```python
from build123d import *

# Parameters (mm, degrees)
SKETCH_1_R          = 12.2
EXTRUDE_1_DEPTH     = 30.8
SKETCH_3_R          = 3.15
EXTRUDE_2_DEPTH     = 2.1
FILLET_1_R          = 0.5
SKETCH_4_R          = 3.225
EXTRUDE_3_DEPTH     = 1.7
SKETCH_6_R          = 1
EXTRUDE_4_DEPTH     = 10
SKETCH_7_R          = 1.1
CUT_EXTRUDE_2_DEPTH = 3


with BuildPart() as part:
    # 草图1 → 凸台-拉伸1 (new body)
    with BuildSketch(Plane(origin=(0, 0, 0), x_dir=(0, 0, -1), z_dir=(1, 0, 0))):
        with Locations(Location((0, 0, 0), (0, 0, 180))):
            Circle(SKETCH_1_R)
    extrude(amount=EXTRUDE_1_DEPTH)

    # 草图3 → 凸台-拉伸2 (add)
    with BuildSketch(Plane(origin=(30.8, 0, 0), x_dir=(0, 0, -1), z_dir=(1, 0, 0))):
        Circle(SKETCH_3_R)
    extrude(amount=EXTRUDE_2_DEPTH)

    # 圆角1
    fillet_1_edges = [part.edges().sort_by_distance(p)[0] for p in [
        (32.9, 0, 3.15),
    ]]
    fillet(fillet_1_edges, radius=FILLET_1_R)

    # 草图4 → 凸台-拉伸3 (add)
    with BuildSketch(Plane.ZY):
        Circle(SKETCH_4_R)
    extrude(amount=EXTRUDE_3_DEPTH)

    # 草图6 → 凸台-拉伸4 (add)
    with BuildSketch(Plane.ZY):
        Circle(SKETCH_6_R)
    extrude(amount=EXTRUDE_4_DEPTH)

    # 草图7 → 切除-拉伸2 (cut)
    with BuildSketch(Plane.ZY):
        with Locations((8.5, 0)):
            Circle(SKETCH_7_R)
        with Locations((-8.5, 0)):
            Circle(SKETCH_7_R)
    extrude(amount=-CUT_EXTRUDE_2_DEPTH, mode=Mode.SUBTRACT)


solid = part.part
```
Geometry check sheet. Reference: the model listing, model coordinates, mm. A direction names the side the tool comes from. Give positions to 0.01 mm unless a question says otherwise; leave off trailing zeros. Order: outer loops, then holes, each group sorted by start corner. A loop starts at its lowest first (then second) coordinate and runs counter-clockwise, first axis right, second up.
1. Release check for a two-part mould opening along Y. For faces 4 (the face through (3, 0, -9)), 5 (the face through (-0.84, -3.15, -0.7)), 6 (the face through (-10, 0, 0)) record: pulls with the +Y half, pulls with the -Y half, needs draft (parallel to the pull), parting line crosses it, or undercut.
2. Section check C-C, the plane x = 2. Enter the section's corners in (y, z), and give its area (3 significant figures).
3. Access from +Z, -Z, +X, -X, +Y, -Y to the whole of each face (thin tool, end or side, straight path). Record for faces 1 (the face through (1.479, -0.421, 9.516)), 2 (the face through (32.9, 0, 0)), 3 (the face through (31.589, -1.917, 2.5)).
4. Section check B-B, the plane z = 0. Enter the section's corners in (x, y) (3 decimals), and give its area (3 significant figures).
5. Gauge pin test, flat ends, axial feed: pin 1 Ø10 at (x, y) = (-2, -5) entering from -Z; pin 2 Ø1.5 at (x, y) = (16, 2.5) entering from -Z; pin 3 Ø4 at (y, z) = (-4.5, 9) entering from +X. Record the tip position at first contact, or that the pin passes through.
6. Thickness scan on L1, parallel to Y at x = 9.5, z = -0.5; L2, parallel to X at y = 6, z = -10.25; L3, parallel to Y at x = 0.8, z = 8.5. Record the ranges inside material, lowest first.
7. Section check A-A, the plane y = 0. Enter the section's corners in (x, z) (3 decimals).
8. Section check D-D, the plane x = 11.5. Enter the section's corners in (y, z).
Values follow:
1. face 4: undercut
1. face 5: parting line crosses it
1. face 6: needs draft
2. outline: circle Ø24.4 at (0, 0); hole circle Ø2.2 at (0, -8.5); hole circle Ø2.2 at (0, 8.5)
2. area: 460 mm2
3. face 1: -X
3. face 2: +Z, -Z, +X, +Y, -Y
3. face 3: +X
4. outline: (-10, -1) - (-1.7, -1) - (-1.7, -3.225) - (0, -3.225) - (0, -12.2) - (30.8, -12.2) - (30.8, -3.15) - (32.4, -3.15) arc R0.5 ccw to (32.9, -2.65) - (32.9, 2.65) arc R0.5 ccw to (32.4, 3.15) - (30.8, 3.15) - (30.8, 12.2) - (0, 12.2) - (0, 3.225) - (-1.7, 3.225) - (-1.7, 1) - (-10, 1) - close
4. area: 792 mm2
5. pin 1: stops at z = -12.19
5. pin 2: stops at z = -12.07
5. pin 3: stops at x = 30.8
6. L1: y = -12.19 to 12.19
6. L2: x = 0 to 30.8
6. L3: y = -8.75 to -1.1, 1.1 to 8.75
7. outline: (-10, -1) - (-1.7, -1) - (-1.7, -3.225) - (0, -3.225) - (0, -7.4) - (3, -7.4) - (3, -9.6) - (0, -9.6) - (0, -12.2) - (30.8, -12.2) - (30.8, -3.15) - (32.4, -3.15) arc R0.5 ccw to (32.9, -2.65) - (32.9, 2.65) arc R0.5 ccw to (32.4, 3.15) - (30.8, 3.15) - (30.8, 12.2) - (0, 12.2) - (0, 9.6) - (3, 9.6) - (3, 7.4) - (0, 7.4) - (0, 3.225) - (-1.7, 3.225) - (-1.7, 1) - (-10, 1) - close
8. outline: circle Ø24.4 at (0, 0)
